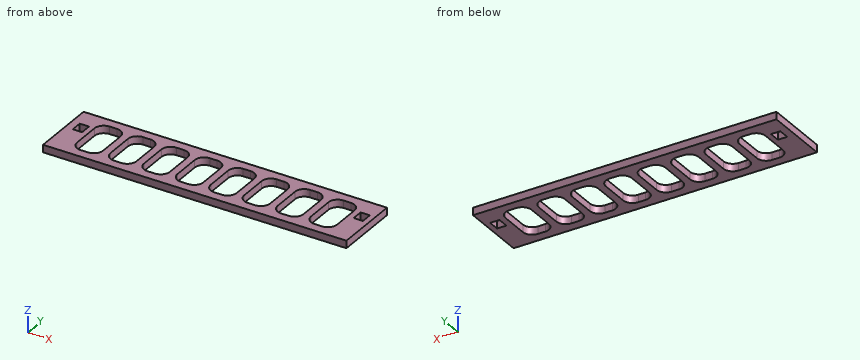
```python
from build123d import *

# Parameters (mm, degrees)
F0_W     = 163.4
F0_H     = 35.05
F0_W_2   = 5
F0_H_2   = 6
F1_DEPTH = 2


with BuildPart() as f1:
    # F0 (on Top) → F1 (new body, symmetric)
    with BuildSketch(Plane.XY):
        with Locations((81.7, 17.525)):
            Rectangle(F0_W, F0_H)
        with BuildLine():
            Line((17.10444, 30.05), (21.10444, 30.05))
            ThreePointArc((21.10444, 30.05), (24.639974, 28.585534), (26.10444, 25.05))
            Line((26.10444, 25.05), (26.10444, 10.05))
            ThreePointArc((26.10444, 10.05), (24.639974, 6.514466), (21.10444, 5.05))
            Line((21.10444, 5.05), (17.10444, 5.05))
            ThreePointArc((17.10444, 5.05), (13.568906, 6.514466), (12.10444, 10.05))
            Line((12.10444, 10.05), (12.10444, 25.05))
            ThreePointArc((12.10444, 25.05), (13.568906, 28.585534), (17.10444, 30.05))
        make_face(mode=Mode.SUBTRACT)
        with BuildLine():
            ThreePointArc((39.10444, 30.05), (42.639974, 28.585534), (44.10444, 25.05))
            Line((44.10444, 25.05), (44.10444, 10.05))
            ThreePointArc((44.10444, 10.05), (42.639974, 6.514466), (39.10444, 5.05))
            Line((39.10444, 5.05), (35.10444, 5.05))
            ThreePointArc((35.10444, 5.05), (31.568906, 6.514466), (30.10444, 10.05))
            Line((30.10444, 10.05), (30.10444, 25.05))
            ThreePointArc((30.10444, 25.05), (31.568906, 28.585534), (35.10444, 30.05))
            Line((35.10444, 30.05), (39.10444, 30.05))
        make_face(mode=Mode.SUBTRACT)
        with Locations((6.666683, 22.05)):
            Rectangle(F0_W_2, F0_H_2, mode=Mode.SUBTRACT)
        with BuildLine():
            ThreePointArc((57.10444, 30.05), (60.639974, 28.585534), (62.10444, 25.05))
            Line((62.10444, 25.05), (62.10444, 10.05))
            ThreePointArc((62.10444, 10.05), (60.639974, 6.514466), (57.10444, 5.05))
            Line((57.10444, 5.05), (53.10444, 5.05))
            ThreePointArc((53.10444, 5.05), (49.568906, 6.514466), (48.10444, 10.05))
            Line((48.10444, 10.05), (48.10444, 25.05))
            ThreePointArc((48.10444, 25.05), (49.568906, 28.585534), (53.10444, 30.05))
            Line((53.10444, 30.05), (57.10444, 30.05))
        make_face(mode=Mode.SUBTRACT)
        with BuildLine():
            ThreePointArc((75.10444, 30.05), (78.639974, 28.585534), (80.10444, 25.05))
            Line((80.10444, 25.05), (80.10444, 10.05))
            ThreePointArc((80.10444, 10.05), (78.639974, 6.514466), (75.10444, 5.05))
            Line((75.10444, 5.05), (71.10444, 5.05))
            ThreePointArc((71.10444, 5.05), (67.568906, 6.514466), (66.10444, 10.05))
            Line((66.10444, 10.05), (66.10444, 25.05))
            ThreePointArc((66.10444, 25.05), (67.568906, 28.585534), (71.10444, 30.05))
            Line((71.10444, 30.05), (75.10444, 30.05))
        make_face(mode=Mode.SUBTRACT)
        with BuildLine():
            ThreePointArc((93.10444, 30.05), (96.639974, 28.585534), (98.10444, 25.05))
            Line((98.10444, 25.05), (98.10444, 10.05))
            ThreePointArc((98.10444, 10.05), (96.639974, 6.514466), (93.10444, 5.05))
            Line((93.10444, 5.05), (89.10444, 5.05))
            ThreePointArc((89.10444, 5.05), (85.568906, 6.514466), (84.10444, 10.05))
            Line((84.10444, 10.05), (84.10444, 25.05))
            ThreePointArc((84.10444, 25.05), (85.568906, 28.585534), (89.10444, 30.05))
            Line((89.10444, 30.05), (93.10444, 30.05))
        make_face(mode=Mode.SUBTRACT)
        with BuildLine():
            ThreePointArc((111.10444, 30.05), (114.639974, 28.585534), (116.10444, 25.05))
            Line((116.10444, 25.05), (116.10444, 10.05))
            ThreePointArc((116.10444, 10.05), (114.639974, 6.514466), (111.10444, 5.05))
            Line((111.10444, 5.05), (107.10444, 5.05))
            ThreePointArc((107.10444, 5.05), (103.568906, 6.514466), (102.10444, 10.05))
            Line((102.10444, 10.05), (102.10444, 25.05))
            ThreePointArc((102.10444, 25.05), (103.568906, 28.585534), (107.10444, 30.05))
            Line((107.10444, 30.05), (111.10444, 30.05))
        make_face(mode=Mode.SUBTRACT)
        with BuildLine():
            ThreePointArc((129.10444, 30.05), (132.639974, 28.585534), (134.10444, 25.05))
            Line((134.10444, 25.05), (134.10444, 10.05))
            ThreePointArc((134.10444, 10.05), (132.639974, 6.514466), (129.10444, 5.05))
            Line((129.10444, 5.05), (125.10444, 5.05))
            ThreePointArc((125.10444, 5.05), (121.568906, 6.514466), (120.10444, 10.05))
            Line((120.10444, 10.05), (120.10444, 25.05))
            ThreePointArc((120.10444, 25.05), (121.568906, 28.585534), (125.10444, 30.05))
            Line((125.10444, 30.05), (129.10444, 30.05))
        make_face(mode=Mode.SUBTRACT)
        with BuildLine():
            ThreePointArc((147.10444, 30.05), (150.639974, 28.585534), (152.10444, 25.05))
            Line((152.10444, 25.05), (152.10444, 10.05))
            ThreePointArc((152.10444, 10.05), (150.639974, 6.514466), (147.10444, 5.05))
            Line((147.10444, 5.05), (143.10444, 5.05))
            ThreePointArc((143.10444, 5.05), (139.568906, 6.514466), (138.10444, 10.05))
            Line((138.10444, 10.05), (138.10444, 25.05))
            ThreePointArc((138.10444, 25.05), (139.568906, 28.585534), (143.10444, 30.05))
            Line((143.10444, 30.05), (147.10444, 30.05))
        make_face(mode=Mode.SUBTRACT)
        with Locations((157.9, 22.05)):
            Rectangle(F0_W_2, F0_H_2, mode=Mode.SUBTRACT)
    extrude(amount=F1_DEPTH, both=True)


solid = f1.part
```
Here's how the part is built. I have some questions about the finished solid (model axes, mm). Give positions to 0.01 mm unless a question says otherwise; leave off trailing zeros. Loops run counter-clockwise (first coordinate to the right, second up) from the corner with the lowest first, then second, coordinate; pieces in that order, holes last. Notation, with made-up numbers: M 78.5,6.5 L 102.5,6.5 A24 cw 102.5,24.5 Z; hole C -10.5,64.25 d1. An arc over 180 degrees is marked long. Put each result on its own line as item: value. Start each with the question number.
(1) I want a section at D-D on x = 139.5. Please give me the cut outline in (y, z).
(2) I want a section at B-B on y = 14.5. State how many separate pieces and enclosed holes the cut face has, then the cut area to 3 significant figures.
(3) I want a section at A-A on x = 108.5. Please give me the cut outline in (y, z).
(4) I need wall thicknesses on line 1 along Y through (x, z) = (129, -0.85). Which ranges of the line are inside material? Lowest first, please. Write a range as [from, to].
Answer block:
1. outline: M 0,-2 L 6.58,-2 L 6.58,2 L 0,2 Z; M 28.52,-2 L 35.05,-2 L 35.05,2 L 28.52,2 Z
2. separate pieces: 9
2. enclosed holes: 0
2. area: 206 mm^2
3. outline: M 0,-2 L 5.05,-2 L 5.05,2 L 0,2 Z; M 30.05,-2 L 35.05,-2 L 35.05,2 L 30.05,2 Z
4. line 1: [0, 5.05], [30.05, 35.05]
